```python
from build123d import *

# Parameters (mm, degrees)
SKETCH1_W               = 76.2
SKETCH1_H               = 69.85
BOSS_EXTRUDE1_DEPTH     = 41.275
SHELL2_T                = 3.175
SKETCH2_W               = 76.2
SKETCH2_H               = 3.175
CUT_EXTRUDE1_DEPTH      = 74.643575755
CUT_EXTRUDE1_DEPTH_BACK = 74.643575755
CUT_EXTRUDE2_REACH      = 75.644
SKETCH4_R               = 2.0828
CUT_EXTRUDE3_DEPTH      = 3.175
SKETCH5_R               = 2.0828
CUT_EXTRUDE4_DEPTH      = 99.629626001
CUT_EXTRUDE4_DEPTH_BACK = 99.629626001


with BuildPart() as part:
    # Sketch1 → Boss-Extrude1 (new body)
    with BuildSketch(Plane(origin=(0, 0, 0), x_dir=(1, 0, 0), z_dir=(0, 1, 0))):
        Rectangle(SKETCH1_W, SKETCH1_H)
    extrude(amount=BOSS_EXTRUDE1_DEPTH)

    # Shell2
    shell2_openings = [part.faces().sort_by_distance(p)[0] for p in [
        (0, 20.6375, 34.925),
    ]]
    offset(amount=SHELL2_T, openings=shell2_openings, kind=Kind.INTERSECTION)

    # Sketch2 → Cut-Extrude1 (cut, two sides)
    with BuildSketch(Plane(origin=(0, 44.45, 0), x_dir=(1, 0, 0), z_dir=(0, 1, 0))) as cut_extrude1_sk:
        with Locations((0, -33.3375)):
            Rectangle(SKETCH2_W, SKETCH2_H)
    extrude(amount=CUT_EXTRUDE1_DEPTH, mode=Mode.SUBTRACT)
    extrude(cut_extrude1_sk.sketch, amount=-CUT_EXTRUDE1_DEPTH_BACK, mode=Mode.SUBTRACT)

    # Sketch3 → Cut-Extrude2 (cut, up to next)
    with BuildSketch(Plane(origin=(0, 44.45, 0), x_dir=(1, 0, 0), z_dir=(0, 1, 0)), mode=Mode.PRIVATE) as cut_extrude2_sk1:
        with BuildLine():
            Line((24.5999, -19.2151), (24.5999, -31.75))
            Line((24.5999, -31.75), (32.2199, -31.75))
            Line((32.2199, -31.75), (32.2199, -19.2151))
            ThreePointArc((32.2199, -19.2151), (28.4099, -15.4051), (24.5999, -19.2151))
        make_face()
    cut_extrude2_tool1 = extrude(cut_extrude2_sk1.sketch, amount=-CUT_EXTRUDE2_REACH, mode=Mode.PRIVATE) & part.part
    add(cut_extrude2_tool1.solids().sort_by_distance((28.4099, 44.45, 23.96308))[0], mode=Mode.SUBTRACT)

    # Sketch4 → Cut-Extrude3 (cut)
    with BuildSketch(Plane.XY.offset(-34.925)):
        with Locations((0, 9.525)):
            Circle(SKETCH4_R)
    extrude(amount=-CUT_EXTRUDE3_DEPTH, mode=Mode.SUBTRACT)

    # Sketch5 → Cut-Extrude4 (cut, two sides)
    with BuildSketch(Plane.ZY.offset(-38.1)) as cut_extrude4_sk:
        with Locations((25.4, 34.925)):
            Circle(SKETCH5_R)
    extrude(amount=CUT_EXTRUDE4_DEPTH, mode=Mode.SUBTRACT)
    extrude(cut_extrude4_sk.sketch, amount=-CUT_EXTRUDE4_DEPTH_BACK, mode=Mode.SUBTRACT)


solid = part.part
```
Verification items for the finished model (mm, model axes). A direction names the side the tool comes from. Coordinates: 2 decimals unless noted, no trailing zeros. Write each loop counter-clockwise with the first axis right and the second up, starting at its lowest first coordinate (ties: lowest second). Pieces come first, ordered by that corner, then holes. Notation, with made-up numbers: M 33.5,47.5 L 64.5,47.5 A26 cw 64.5,70.5 Z; hole C -24.75,-20.75 d4. An arc over 180 degrees is marked long. One line per item, written item: value.
Item 1: Section check D-D, the plane y = 1. Record the boundary of the cut face in (x, z) (3 decimals), plus the area to 3 significant figures.
Check sheet entries:
outline: M -41.275,-38.1 L 41.275,-38.1 L 41.275,34.925 L 38.1,34.925 L 38.1,-34.925 L -38.1,-34.925 L -38.1,34.925 L -41.275,34.925 Z
area: 706 mm^2
Item 2: Mould release check, pull along Y, two halves, no side actions. Record for faces 1 (the flat face through (-38.1, 20, 0)), 2 (the flat face through (-1, 44.45, -2)), 3 (the flat face through (-1, -2, 31.75)), 4 (the flat face through (-1, -3.175, -2)): pulls with the +Y half, pulls with the -Y half, needs draft (parallel to the pull), parting line crosses it, or undercut.
Check sheet entries:
face 1: undercut
face 2: pulls with the +Y half
face 3: needs draft
face 4: pulls with the -Y half
Item 3: Scan lines: line 1 along X through (y, z) = (26, 8.5) (3 decimals); line 2 along Y through (x, z) = (0, -35.95) (3 decimals); line 3 along Y through (x, z) = (13, -26) (3 decimals). Record each from-to range of solid material in increasing order.
Check sheet entries:
line 1: x = -41.275 to -38.1, 38.1 to 41.275
line 2: y = -3.175 to 7.442, 11.608 to 44.45
line 3: y = -3.175 to 0, 41.275 to 44.45
Item 4: Access from +Z, -Z, +X, -X, +Y, -Y to the whole of each face (thin tool, end or side, straight path). Record for faces 5 (the flat face through (38.1, 21, 0)), 6 (the flat face through (-41.275, 20, -1)), 7 (the cylindrical face through (28.494, 42.885, 15.406)), 8 (the flat face through (-7, 43, 31.75)).
Check sheet entries:
face 5: +Z
face 6: +Z, -Z, -X, +Y, -Y
face 7: +Z, +Y
face 8: +Z, +Y, -Y
Item 5: Section check C-C, the plane x = 16.5. Record the boundary of the cut face in (y, z) (3 decimals).
Check sheet entries:
outline: M -3.175,-38.1 L 44.45,-38.1 L 44.45,31.75 L 41.275,31.75 L 41.275,-34.925 L 0,-34.925 L 0,31.75 L -3.175,31.75 Z
Item 6: Gauge pin test, flat ends, axial feed: pin 1 Ø4 at (x, y) = (-15, 32.5) entering from +Z (3 decimals); pin 2 Ø4 at (x, z) = (29, 24.5) entering from +Y; pin 3 Ø3.5 at (x, y) = (0, 9.525) entering from -Z; pin 4 Ø2.5 at (x, y) = (34.5, 43.5) entering from +Z. Record the tip position at first contact, or that the pin passes through.
Check sheet entries:
pin 1: stops at z = -34.925
pin 2: stops at y = 0
pin 3: passes through
pin 4: stops at z = 31.75
Item 7: Section check A-A, the plane z = 25.4. Record the boundary of the cut face in (x, y) (3 decimals), plus the area to 3 significant figures.
Check sheet entries:
outline: M -41.275,-3.175 L 41.275,-3.175 L 41.275,32.842 L 38.1,32.842 L 38.1,0 L -38.1,0 L -38.1,32.842 L -41.275,32.842 Z; M -41.275,37.008 L -38.1,37.008 L -38.1,41.275 L 24.6,41.275 L 24.6,44.45 L -41.275,44.45 Z; M 32.22,41.275 L 38.1,41.275 L 38.1,37.008 L 41.275,37.008 L 41.275,44.45 L 32.22,44.45 Z
area: 736 mm^2
Item 8: Section check B-B, the plane z = 2. Record the boundary of the cut face in (x, y) (3 decimals), plus the area to 3 significant figures.
Check sheet entries:
outline: M -41.275,-3.175 L 41.275,-3.175 L 41.275,44.45 L -41.275,44.45 Z; hole M -38.1,0 L 38.1,0 L 38.1,41.275 L -38.1,41.275 Z
area: 786 mm^2
